from build123d import *

# Parameters (mm, degrees)
SKETCH1_R           = 15
BOSS_EXTRUDE1_DEPTH = 14.75
CUT_EXTRUDE1_DEPTH  = 15.75
CIRPATTERN1_COUNT   = 16
CUT_EXTRUDE2_DEPTH  = 15.75


with BuildPart() as part:
    # Sketch1 → Boss-Extrude1 (new body)
    with BuildSketch(Plane.XY):
        Circle(SKETCH1_R)
    extrude(amount=BOSS_EXTRUDE1_DEPTH)

    # Sketch2 → Cut-Extrude1 (cut, through all)
    with BuildSketch(Plane.XY.offset(14.75)):
        with BuildLine():
            ThreePointArc((-1, 10.95445115), (0, 11), (1, 10.95445115))
            ThreePointArc((1, 10.95445115), (1.384034944, 13.063153145), (2.7, 14.754999153))
            ThreePointArc((2.7, 14.754999153), (0, 15), (-2.7, 14.754999153))
            ThreePointArc((-2.7, 14.754999153), (-1.384034944, 13.063153145), (-1, 10.95445115))
        make_face()
    cut_extrude1 = extrude(amount=-CUT_EXTRUDE1_DEPTH, mode=Mode.SUBTRACT)

    # CirPattern1: Cut-Extrude1 ×16 about axis
    cirpattern1_axis = Axis((0, 0, 0), (0, 0, 1))
    for i in range(1, CIRPATTERN1_COUNT):
        add(cut_extrude1.rotate(cirpattern1_axis, i * 360 / CIRPATTERN1_COUNT), mode=Mode.SUBTRACT)

    # Sketch3 → Cut-Extrude2 (cut, through all)
    with BuildSketch(Plane.XY.offset(14.75)):
        with BuildLine():
            Line((2.0058, 1.47542074), (2.0058, -1.47542074))
            ThreePointArc((2.0058, -1.47542074), (-2.49, 0), (2.0058, 1.47542074))
        make_face()
    extrude(amount=-CUT_EXTRUDE2_DEPTH, mode=Mode.SUBTRACT)


solid = part.part
The listing builds one solid part. Answer for the finished solid, in the listing's coordinates (mm). Round coordinates to 2 decimals unless told otherwise and drop trailing zeros. Write each loop counter-clockwise with the first axis right and the second up, starting at its lowest first coordinate (ties: lowest second). Pieces come first, ordered by that corner, then holes. Notation, with made-up numbers: M 53,81 L 80,81 A30 cw 80,108 Z; hole C 30,76.5 d2. An arc over 180 degrees is marked long. Write each question's results on one line, items separated by ' | '. Start each with the question number.
(1) The part is cut by section C-C, the plane y = -6.25. Write down the section's boundary in (x, z).
(2) The part is cut by section A-A, the plane x = 0. Write down the section's boundary in (y, z), and give its area (3 significant figures).
(3) Each of these flat-tipped pins is pushed along its axis until it touches: P1, Ø3, axis at y = -0.5, z = 2, coming from the -X side; P2, Ø8, axis at y = 7, z = 6, coming from the +X side; P3, Ø3, axis at x = -11.5, z = 8.5, coming from the +Y side. Where does it stop, or does it pass through?
(4) Determine the mould class of faces 1 (the flat face through (-3, 0, 14.75)), 2 (the cylindrical face through (-3.72, -12.63, 7.48)), 3 (the cylindrical face through (10.16, 4.22, 7.48)) for opening direction X: +X half, -X half, draft (parallel to the pull), parting line (faces both ways), or undercut.
(5) Find the intervals of material crossed by line 1 (Y direction, x = 0, z = 8.75); line 2 (Y direction, x = -10.75, z = 1.5) (3 decimals); line 3 (X direction, y = 0, z = 4.5), in increasing order.
(6) The part is cut by section B-B, the plane y = 0. Write down the section's boundary in (x, z), and give its area (3 significant figures).
Worked answers:
1) outline: M -11.51,0 L 11.51,0 L 11.51,14.75 L -11.51,14.75 Z
2) outline: M -11,0 L -2.49,0 L -2.49,14.75 L -11,14.75 Z; M 2.49,0 L 11,0 L 11,14.75 L 2.49,14.75 Z | area: 251 mm²
3) P1: stops at x = -14.06 | P2: stops at x = 14.7 | P3: stops at y = 8.55
4) face 1: draft | face 2: undercut | face 3: undercut
5) line 1: y = -11 to -2.49, 2.49 to 11 | line 2: y = -8.425 to -5.615, -3.379 to 3.379, 5.615 to 8.425 | line 3: x = -11 to -2.49, 2.01 to 11
6) outline: M -11,0 L -2.49,0 L -2.49,14.75 L -11,14.75 Z; M 2.01,0 L 11,0 L 11,14.75 L 2.01,14.75 Z | area: 258 mm²
